The listing builds one solid part. Answer for the finished solid, in the listing's coordinates (mm). Face numbers are marked on the shaded views. Give positions to 0.01 mm unless a question says otherwise; leave off trailing zeros. Order: outer loops, then holes, each group sorted by start corner. A loop starts at its lowest first (then second) coordinate and runs counter-clockwise, first axis right, second up. Notation, with made-up numbers: (37, 27) - (43, 27) arc R14 ccw to (43, 43) - close; hole circle Ø4 at (5, -6.5). An arc over 180 degrees is marked (long way). Answer as a JSON object with one key per item and string values. Group by question number.
Q1. A cutting plane is placed at A-A, the plane x = 0. Give the vertices of the cut face in (y, z), and give its area (3 significant figures).
Q2. Consider line 1 (Z direction, x = -45, y = 27); line 2 (Y direction, x = 0, z = 1.4); line 3 (Z direction, x = -45, y = 21) (3 decimals). Determine where each line is inside the solid, lowest interval first.
Q3. A cutting plane is placed at C-C, the plane z = -20.4. Give the vertices of the cut face in (x, y) (3 decimals).
Q4. A cutting plane is placed at B-B, the plane z = -7. Give the vertices of the cut face in (x, y), and give its area (3 significant figures).
Q5. The mould has two halves that part along X. Classify the marked faces 1, 2 and 3: released by +X, released by -X, zero draft, split by the parting line, or undercut.
Q6. Given pin 1 (2 mm diameter, centred on x = 30, y = 11, fed in from -Z); pin 2 (5.5 mm diameter, centred on x = 46, z = -18, fed in from -Y); pin 3 (3 mm diameter, centred on x = 30.5, z = -14.5, fed in from -Y), each flat-ended and moving along its own axis, determine where each tip first touches the part or whether it passes through.
Q7. A cutting plane is placed at D-D, the plane y = 0. Give the vertices of the cut face in (x, z).
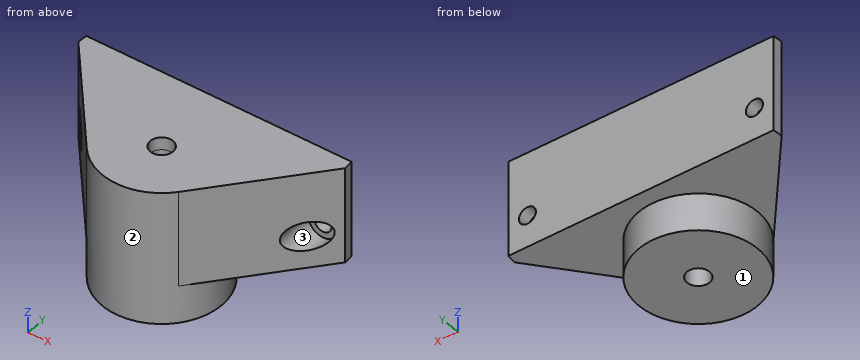
from build123d import *
from OCP.BRepFilletAPI import BRepFilletAPI_MakeChamfer

# Parameters (mm, degrees)
SKETCH1_R               = 23.7
SKETCH1_R_2             = 18.7
BOSS_EXTRUDE1_DEPTH     = 48
BOSS_EXTRUDE2_START     = 5
SKETCH1_3_R             = 23.7
SKETCH1_3_R_2           = 18.7
SKETCH1_3_R_3           = 15.5
SKETCH1_3_R_4           = 6.5
BOSS_EXTRUDE2_DEPTH     = 5
BOSS_EXTRUDE3_DEPTH     = 38.1
F_1_4_CLEARANCE_HOLE1_D = 6.7564
SKETCH9_R               = 5.715
CUT_EXTRUDE1_DEPTH      = 89.454226705
CHAMFER1_SIZE           = 5
CHAMFER1_SIZE2          = 3.549039071
SKETCH10_R              = 18.7
SKETCH10_R_2            = 4.5
BOSS_EXTRUDE4_DEPTH     = 48
SKETCH10_2_R            = 4.5
CUT_EXTRUDE2_DEPTH      = 78.473312523


with BuildPart() as part:
    # Sketch1 → Boss-Extrude1 (new body)
    with BuildSketch(Plane.XY):
        Circle(SKETCH1_R)
        Circle(SKETCH1_R_2, mode=Mode.SUBTRACT)
    extrude(amount=-BOSS_EXTRUDE1_DEPTH)

    # Sketch1<3> → Boss-Extrude2 (add)
    # profile 1 of 4: a face of its own
    with BuildSketch(Plane.XY.offset(BOSS_EXTRUDE2_START)):
        Circle(SKETCH1_3_R)
        Circle(SKETCH1_3_R_2, mode=Mode.SUBTRACT)
    # profile 2 of 4: a face of its own
    with BuildSketch(Plane.XY.offset(BOSS_EXTRUDE2_START)):
        Circle(SKETCH1_3_R_2)
        Circle(SKETCH1_3_R_3, mode=Mode.SUBTRACT)
    # profile 3 of 4: a face of its own
    with BuildSketch(Plane.XY.offset(BOSS_EXTRUDE2_START)):
        Circle(SKETCH1_3_R_3)
        with Locations((0, 7.5)):
            Circle(SKETCH1_3_R_4, mode=Mode.SUBTRACT)
    # profile 4 of 4: a face of its own
    with BuildSketch(Plane.XY.offset(BOSS_EXTRUDE2_START)):
        with Locations((0, 7.5)):
            Circle(SKETCH1_3_R_4)
    extrude(amount=-BOSS_EXTRUDE2_DEPTH)

    # Sketch5 → Boss-Extrude3 (add)
    with BuildSketch(Plane.XY.offset(5)):
        with BuildLine():
            Line((56.111141692, 30), (-56.111141692, 30))
            Line((-56.111141692, 30), (-18.155253302, -15.23406635))
            ThreePointArc((-18.155253302, -15.23406635), (-8.105877397, 22.270715113), (23.7, 0))
            ThreePointArc((23.7, 0), (22.270715113, -8.105877397), (18.155253302, -15.23406635))
            Line((18.155253302, -15.23406635), (56.111141692, 30))
        make_face()
    extrude(amount=-BOSS_EXTRUDE3_DEPTH)

    # 1/4 Clearance Hole1 (through all)
    with Locations(Plane(origin=(0, 30, 0), x_dir=(1, 0, 0), z_dir=(0, 1, 0))):
        with Locations((-45, 20.4), (45, 20.4)):
            Hole(F_1_4_CLEARANCE_HOLE1_D / 2)

    # Sketch9 → Cut-Extrude1 (cut, through all)
    with BuildSketch(Plane(origin=(0, 25, 0), x_dir=(1, 0, 0), z_dir=(0, 1, 0))):
        with Locations(Location((-45, 20.4, 0), (0, 0, 180))):
            Circle(SKETCH9_R)
        with Locations(Location((45, 20.4, 0), (0, 0, 180))):
            Circle(SKETCH9_R)
    extrude(amount=-CUT_EXTRUDE1_DEPTH, mode=Mode.SUBTRACT)

    # Chamfer1: one chamfer whose edges measure the first distance from different faces: ONE call of the kernel's chamfer builder (chamfer() names one face for all edges)
    chamfer1_edges_1 = [part.edges().sort_by_distance(p)[0] for p in [
        (56.111141692, 30, -14.05),
    ]]
    chamfer1_side_1 = [part.faces().sort_by_distance(p)[0] for p in [
        (36.532384477, 6.666945749, -13.565030067),
    ]]
    chamfer1_edges_2 = [part.edges().sort_by_distance(p)[0] for p in [
        (-56.111141692, 30, -14.05),
    ]]
    chamfer1_side_2 = [part.faces().sort_by_distance(p)[0] for p in [
        (-36.532384477, 6.666945749, -13.565030067),
    ]]
    chamfer1 = BRepFilletAPI_MakeChamfer(part.part.solid().wrapped)
    for e in chamfer1_edges_1:
        chamfer1.Add(CHAMFER1_SIZE, CHAMFER1_SIZE2, e.wrapped, chamfer1_side_1[0].wrapped)  # the first distance lies on this face
    for e in chamfer1_edges_2:
        chamfer1.Add(CHAMFER1_SIZE, CHAMFER1_SIZE2, e.wrapped, chamfer1_side_2[0].wrapped)  # the first distance lies on this face
    add(Compound.cast(chamfer1.Shape()), mode=Mode.REPLACE)

    # Sketch10 → Boss-Extrude4 (add)
    with BuildSketch(Plane(origin=(0, 0, 0), x_dir=(-1, 0, 0), z_dir=(0, 0, -1))):
        Circle(SKETCH10_R)
        with Locations(Location((0, 0, 0), (0, 0, 180))):
            Circle(SKETCH10_R_2, mode=Mode.SUBTRACT)
    extrude(amount=BOSS_EXTRUDE4_DEPTH)

    # Sketch10<2> → Cut-Extrude2 (cut, through all)
    with BuildSketch(Plane(origin=(0, 0, 0), x_dir=(-1, 0, 0), z_dir=(0, 0, -1))):
        with Locations(Location((0, 0, 0), (0, 0, 180))):
            Circle(SKETCH10_2_R)
    extrude(amount=-CUT_EXTRUDE2_DEPTH, mode=Mode.SUBTRACT)


solid = part.part
Reply:
{
 "1": {"outline": "(-23.7, -48) - (-4.5, -48) - (-4.5, 5) - (-23.7, 5) - close; (4.5, -48) - (23.7, -48) - (23.7, -33.1) - (30, -33.1) - (30, 5) - (4.5, 5) - close", "area": "2,280 mm^2"},
 "2": {"line 1": "z = -33.1 to -23.78, -17.02 to 5", "line 2": "y = -23.7 to -4.5, 4.5 to 30", "line 3": "z = -33.1 to -26.115, -14.685 to 5"},
 "3": {"outline": "(-52.897, 26.17) - (-50.715, 23.569) - (-50.715, 25) - (-48.378, 25) - (-48.378, 30) - (-52.562, 30) - close; (-41.622, 25) - (-39.285, 25) - (-39.285, 9.947) - (-18.155, -15.234) arc R23.7 ccw to (18.155, -15.234) - (39.285, 9.947) - (39.285, 25) - (41.622, 25) - (41.622, 30) - (-41.622, 30) - close; (48.378, 25) - (50.715, 25) - (50.715, 23.569) - (52.897, 26.17) - (52.562, 30) - (48.378, 30) - close; hole circle Ø9 at (0, 0)"},
 "4": {"outline": "(-52.9, 26.17) - (-18.16, -15.23) arc R23.7 ccw to (18.16, -15.23) - (52.9, 26.17) - (52.56, 30) - (-52.56, 30) - close; hole circle Ø9 at (0, 0)", "area": "3,500 mm^2"},
 "5": {"face 1": "zero draft", "face 2": "split by the parting line", "face 3": "undercut"},
 "6": {"pin 1": "stops at z = -33.1", "pin 2": "stops at y = 25", "pin 3": "stops at y = -2.31"},
 "7": {"outline": "(-30.94, -33.1) - (-23.7, -33.1) - (-23.7, -48) - (-4.5, -48) - (-4.5, 5) - (-30.94, 5) - close; (4.5, -48) - (23.7, -48) - (23.7, -33.1) - (30.94, -33.1) - (30.94, 5) - (4.5, 5) - close"}
}
